Read the model definition and answer for the solid it produces. Units are mm, in the model's axes. A direction names the side the tool comes from. Coordinates: 2 decimals unless noted, no trailing zeros. Loops run counter-clockwise (first coordinate to the right, second up) from the corner with the lowest first, then second, coordinate; pieces in that order, holes last.
from build123d import *

# Parameters (mm, degrees)
F1_DEPTH = 3.175


with BuildPart() as f1:
    # F0 (on Top) → F1 (new body)
    with BuildSketch(Plane.XY):
        Polygon((0, 9.071429), (0, 0), (123.825, 0), (123.825, 9.071429), (127, 9.071429), (127, 18.142857), (123.825, 18.142857), (123.825, 27.214286), (127, 27.214286), (127, 36.285714), (123.825, 36.285714), (123.825, 45.357143), (127, 45.357143), (127, 54.428571), (123.825, 54.428571), (123.825, 63.5), (0, 63.5), (0, 54.428571), (3.175, 54.428571), (3.175, 45.357143), (0, 45.357143), (0, 36.285714), (3.175, 36.285714), (3.175, 27.214286), (0, 27.214286), (0, 18.142857), (3.175, 18.142857), (3.175, 9.071429), align=None)
    extrude(amount=F1_DEPTH)


solid = f1.part
Item 1: A cutting plane is placed at B-B on y = 50. Determine the outline of the cut face in (x, z) (3 decimals).
Numbers:
outline: (3.175, 0) - (127, 0) - (127, 3.175) - (3.175, 3.175) - close
Item 2: Which of the six approach directions +Z, -Z, +X, -X, +Y, -Y give full straight-line access (tool end or side, diameter ignored) to faces 1 (the face through (63, 32, 3.175)), 2 (the face through (3.175, 14, 2)), 3 (the face through (123.825, 59, 2)), 4 (the face through (125, 18.143, 2))?
Numbers:
face 1: +Z, +X, -X, +Y, -Y
face 2: +Z, -Z, -X
face 3: +Z, -Z, +X, +Y
face 4: +Z, -Z, +X
Item 3: A cutting plane is placed at A-A on z = 1.5. Determine the outline of the cut face in (x, y) (3 decimals), then the cut area to 3 significant figures.
Numbers:
outline: (0, 0) - (123.825, 0) - (123.825, 9.071) - (127, 9.071) - (127, 18.143) - (123.825, 18.143) - (123.825, 27.214) - (127, 27.214) - (127, 36.286) - (123.825, 36.286) - (123.825, 45.357) - (127, 45.357) - (127, 54.429) - (123.825, 54.429) - (123.825, 63.5) - (0, 63.5) - (0, 54.429) - (3.175, 54.429) - (3.175, 45.357) - (0, 45.357) - (0, 36.286) - (3.175, 36.286) - (3.175, 27.214) - (0, 27.214) - (0, 18.143) - (3.175, 18.143) - (3.175, 9.071) - (0, 9.071) - close
area: 7,860 mm2
Item 4: Find the intervals of material crossed by line 1 along X through (y, z) = (32, 2.8) (3 decimals); line 2 along X through (y, z) = (45, 1.75) (3 decimals), in increasing order.
Numbers:
line 1: x = 3.175 to 127
line 2: x = 0 to 123.825
Item 5: Given pin 1 (1 mm diameter, centred on x = 125, z = 2, fed in from -Y); pin 2 (1.6 mm diameter, centred on y = 12, z = 1, fed in from -X) (3 decimals); pin 3 (1.6 mm diameter, centred on x = 125, z = 1, fed in from +Y), each flat-ended and moving along its own axis, determine where each tip first touches the part or whether it passes through.
Numbers:
pin 1: stops at y = 9.07
pin 2: stops at x = 3.175
pin 3: stops at y = 54.43
